Part model, mm, in its own coordinate system. A direction names the side the tool comes from. Round coordinates to 2 decimals unless told otherwise and drop trailing zeros.
```python
from build123d import *

# Parameters (mm, degrees)
SKETCH_1_W             = 23.5
SKETCH_1_H             = 12
EXTRUDE_1_DEPTH        = 254.5
HOLE_WIZARD_M6_1_D     = 5
HOLE_WIZARD_M6_1_DEPTH = 19
HOLE_WIZARD_M6_1_TIP   = 1.502151548
HOLE_WIZARD_M6_2_D     = 5
HOLE_WIZARD_M6_2_DEPTH = 19
HOLE_WIZARD_M6_2_TIP   = 1.502151548
HOLE_WIZARD_M4_1_D     = 3.3
HOLE_WIZARD_M4_1_DEPTH = 11.5
HOLE_WIZARD_M4_1_TIP   = 0.991420021


with BuildPart() as part:
    # 草图1 → 凸台-拉伸1 (new, symmetric)
    with BuildSketch(Plane(origin=(0, 0, 0), x_dir=(0, 0, -1), z_dir=(1, 0, 0))):
        Polygon((-15, 15), (-11.5, 15), (-11.5, 13.5), (-11, 13.5), (-11, 12), (-9.5, 12), (-9.5, 15), (-8, 15), (-8, 12.5), (-5, 12.5), (-5, 15), (5, 15), (5, 12.5), (8, 12.5), (8, 15), (9.5, 15), (9.5, 12), (11, 12), (11, 13.5), (11.5, 13.5), (11.5, 15), (15, 15), (15, 8), (12.5, 8), (12.5, 5), (15, 5), (15, -5), (12.5, -5), (12.5, -8), (15, -8), (15, -15), (11.5, -15), (11.5, -13.5), (11, -13.5), (11, -12), (9.5, -12), (9.5, -15), (8, -15), (8, -12.5), (5, -12.5), (5, -15), (-5, -15), (-5, -12.5), (-8, -12.5), (-8, -15), (-9.5, -15), (-9.5, -12), (-11, -12), (-11, -13.5), (-11.5, -13.5), (-11.5, -15), (-15, -15), align=None)
        with BuildLine():
            Line((12, -10.5), (12, -8.5))
            ThreePointArc((12, -8.5), (11.853553391, -8.146446609), (11.5, -8))
            Line((11.5, -8), (-11.5, -8))
            ThreePointArc((-11.5, -8), (-11.853553391, -8.146446609), (-12, -8.5))
            Line((-12, -8.5), (-12, -10.5))
            ThreePointArc((-12, -10.5), (-11.853553391, -10.853553391), (-11.5, -11))
            Line((-11.5, -11), (11.5, -11))
            ThreePointArc((11.5, -11), (11.853553391, -10.853553391), (12, -10.5))
        make_face(mode=Mode.SUBTRACT)
        with BuildLine():
            Line((-11.5, 11), (11.5, 11))
            ThreePointArc((11.5, 11), (11.853553391, 10.853553391), (12, 10.5))
            Line((12, 10.5), (12, 8.5))
            ThreePointArc((12, 8.5), (11.853553391, 8.146446609), (11.5, 8))
            Line((11.5, 8), (-11.5, 8))
            ThreePointArc((-11.5, 8), (-11.853553391, 8.146446609), (-12, 8.5))
            Line((-12, 8.5), (-12, 10.5))
            ThreePointArc((-12, 10.5), (-11.853553391, 10.853553391), (-11.5, 11))
        make_face(mode=Mode.SUBTRACT)
        Rectangle(SKETCH_1_W, SKETCH_1_H, mode=Mode.SUBTRACT)
    extrude(amount=EXTRUDE_1_DEPTH, both=True)

    # M6 螺纹孔1
    with Locations(Plane(origin=(0, 0, -15), x_dir=(-1, 0, 0), z_dir=(0, 0, -1))):
        with Locations((16.5, 0), (1.5, 0), (-219.5, 0), (-234.5, 0)):
            Hole(HOLE_WIZARD_M6_1_D / 2, depth=HOLE_WIZARD_M6_1_DEPTH)
            with Locations((0, 0, -(HOLE_WIZARD_M6_1_DEPTH + HOLE_WIZARD_M6_1_TIP / 2))):  # 118° drill point
                Cone(0, HOLE_WIZARD_M6_1_D / 2, HOLE_WIZARD_M6_1_TIP, mode=Mode.SUBTRACT)

    # M6 螺纹孔2
    with Locations(Plane(origin=(0, -15, 0), x_dir=(-1, 0, 0), z_dir=(0, -1, 0))):
        with Locations((-219.5, 0), (-234.5, 0), (234.5, 0), (219.5, 0)):
            Hole(HOLE_WIZARD_M6_2_D / 2, depth=HOLE_WIZARD_M6_2_DEPTH)
            with Locations((0, 0, -(HOLE_WIZARD_M6_2_DEPTH + HOLE_WIZARD_M6_2_TIP / 2))):  # 118° drill point
                Cone(0, HOLE_WIZARD_M6_2_D / 2, HOLE_WIZARD_M6_2_TIP, mode=Mode.SUBTRACT)

    # M4 螺纹孔1
    with Locations(Plane(origin=(0, -15, 0), x_dir=(-1, 0, 0), z_dir=(0, -1, 0))):
        with Locations((-131, 0), (51.5, 0)):
            Hole(HOLE_WIZARD_M4_1_D / 2, depth=HOLE_WIZARD_M4_1_DEPTH)
            with Locations((0, 0, -(HOLE_WIZARD_M4_1_DEPTH + HOLE_WIZARD_M4_1_TIP / 2))):  # 118° drill point
                Cone(0, HOLE_WIZARD_M4_1_D / 2, HOLE_WIZARD_M4_1_TIP, mode=Mode.SUBTRACT)


solid = part.part
```
Q1. Drop flat-ended pins along their axis: pin 1 (1.5 mm diameter, centred on x = 109, y = -6, fed in from -Z); pin 2 (3 mm diameter, centred on x = 219.5, y = 0, fed in from -Z); pin 3 (1 mm diameter, centred on x = -87, z = 7, fed in from +Y). Give the stop position or say it passes through.
Values follow:
pin 1: stops at z = -12.5
pin 2: stops at z = 11.75
pin 3: stops at y = 12.5
Q2. Cut at A-A on x = 139. State how many separate pieces and enclosed holes the cut face has, plus the area to 3 significant figures.
Values follow:
separate pieces: 1
enclosed holes: 3
area: 408 mm2
Q3. Mould opens along Z. For faces 3 (the flat face through (4, 0, 15)), 4 (the flat face through (4, 8, 0)), 5 (the flat face through (-254.5, 7, 0)), 6 (the flat face through (4, -8, 0)) say: +Z half, -Z half, draft (parallel to the pull), parting line (faces both ways), or undercut.
Values follow:
face 3: +Z half
face 4: undercut
face 5: draft
face 6: undercut
Q4. Which spindle directions (+Z, -Z, +X, -X, +Y, -Y) get a long thin tool onto all of the face, cutting with end or side? Do faces 1 (the flat face through (4, 0, -15)), 2 (the flat face through (4, 6, 0)). Say none if no direction does.
Values follow:
face 1: -Z, +X, -X, +Y, -Y
face 2: +X, -X
Q5. Wall check: L1, parallel to Y at x = -181, z = -2.75; L2, parallel to Y at x = 169, z = -13.5; L3, parallel to Y at x = 19.5, z = -10.25. Give the ranges that are in metal, low to high.
Values follow:
L1: y = -15 to -11, -8 to -6, 6 to 8, 11 to 15
L2: y = -15 to -8, -5 to 5, 8 to 15
L3: y = -12 to -11, -8 to -6, 6 to 8, 11 to 12
